The model under review builds one solid part; all positions refer to its coordinate system, in mm. Give positions to 0.01 mm unless a question says otherwise; leave off trailing zeros. Order: outer loops, then holes, each group sorted by start corner. A loop starts at its lowest first (then second) coordinate and runs counter-clockwise, first axis right, second up. Notation, with made-up numbers: (80.25, 50.5) -> (113.25, 50.5) arc R36 ccw to (113.25, 88.5) -> close; hole circle Ø9 at (-29, -3). An arc over 180 degrees is marked (long way). Use one line per item in the form item = value.
```python
from build123d import *

# Parameters (mm, degrees)
SKETCH1_W            = 20.32
SKETCH1_H            = 15.24
BOSS_EXTRUDE1_DEPTH  = 1.651
SKETCH3_W            = 3.048
SKETCH3_H            = 3.81
BOSS_EXTRUDE3_DEPTH  = 0.6604
SKETCH4_R            = 1.524
BOSS_EXTRUDE4_DEPTH  = 0.7366
SKETCH7_R            = 0.3937
CUT_EXTRUDE2_DEPTH   = 2.651
LPATTERN2_COUNT      = 8
LPATTERN2_PITCH      = 2.54
LPATTERN2_COUNT_DIR2 = 2
LPATTERN2_PITCH_DIR2 = 12.7
CUT_EXTRUDE3_REACH   = 3.651
SKETCH8_R            = 0.3937


with BuildPart() as part:
    # Sketch1 → Boss-Extrude1 (new body)
    with BuildSketch(Plane(origin=(0, 0, 0), x_dir=(1, 0, 0), z_dir=(0, 1, 0))):
        Rectangle(SKETCH1_W, SKETCH1_H)
    extrude(amount=BOSS_EXTRUDE1_DEPTH)

    # Sketch3 → Boss-Extrude3 (add)
    with BuildSketch(Plane(origin=(0, 1.651, 0), x_dir=(1, 0, 0), z_dir=(0, 1, 0))):
        with Locations((7.62, -2.921)):
            Rectangle(SKETCH3_W, SKETCH3_H)
    extrude(amount=BOSS_EXTRUDE3_DEPTH)

    # Sketch4 → Boss-Extrude4 (add)
    with BuildSketch(Plane(origin=(0, 2.3114, 0), x_dir=(1, 0, 0), z_dir=(0, 1, 0))):
        with Locations((7.62, -2.921)):
            Circle(SKETCH4_R)
        Polygon((7.8105, -2.7305), (8.636, -2.7305), (8.636, -3.1115), (7.8105, -3.1115), (7.8105, -3.937), (7.4295, -3.937), (7.4295, -3.1115), (6.604, -3.1115), (6.604, -2.7305), (7.4295, -2.7305), (7.4295, -1.905), (7.8105, -1.905), align=None, mode=Mode.SUBTRACT)
    extrude(amount=BOSS_EXTRUDE4_DEPTH)

    # Sketch7 → Cut-Extrude2 (cut, through all)
    with BuildSketch(Plane(origin=(0, 1.651, 0), x_dir=(1, 0, 0), z_dir=(0, 1, 0))):
        with Locations((-8.89, -6.35)):
            Circle(SKETCH7_R)
    cut_extrude2 = extrude(amount=-CUT_EXTRUDE2_DEPTH, mode=Mode.SUBTRACT)

    # LPattern2: Cut-Extrude2 8 × 2
    with Locations(*[(i * LPATTERN2_PITCH, 0, -j * LPATTERN2_PITCH_DIR2) for i in range(LPATTERN2_COUNT) for j in range(LPATTERN2_COUNT_DIR2) if (i, j) != (0, 0)]):
        add(cut_extrude2, mode=Mode.SUBTRACT)

    # Sketch8 → Cut-Extrude3 (cut, up to next)
    with BuildSketch(Plane(origin=(0, 1.651, 0), x_dir=(1, 0, 0), z_dir=(0, 1, 0)), mode=Mode.PRIVATE) as cut_extrude3_sk1:
        with Locations((8.89, 3.81)):
            Circle(SKETCH8_R)
    cut_extrude3_tool1 = extrude(cut_extrude3_sk1.sketch, amount=-CUT_EXTRUDE3_REACH, mode=Mode.PRIVATE) & part.part
    add(cut_extrude3_tool1.solids().sort_by_distance((8.89, 1.651, -3.81))[0], mode=Mode.SUBTRACT)
    # Sketch8 → Cut-Extrude3 (cut, up to next)
    with BuildSketch(Plane(origin=(0, 1.651, 0), x_dir=(1, 0, 0), z_dir=(0, 1, 0)), mode=Mode.PRIVATE) as cut_extrude3_sk2:
        with Locations((8.89, 1.27)):
            Circle(SKETCH8_R)
    cut_extrude3_tool2 = extrude(cut_extrude3_sk2.sketch, amount=-CUT_EXTRUDE3_REACH, mode=Mode.PRIVATE) & part.part
    add(cut_extrude3_tool2.solids().sort_by_distance((8.89, 1.651, -1.27))[0], mode=Mode.SUBTRACT)


solid = part.part
```
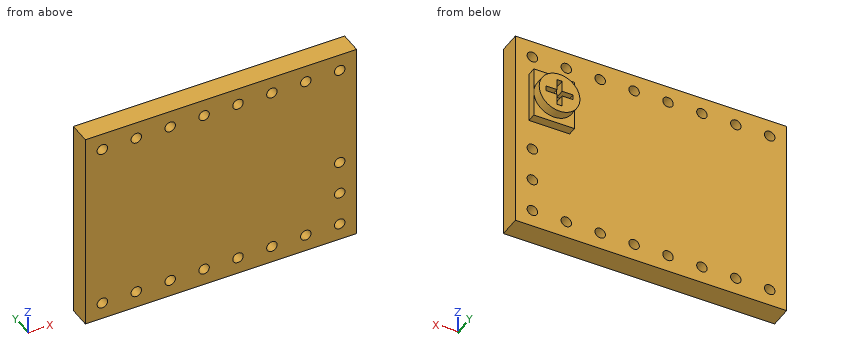
1. Add section A-A on z = -3.81. Give the boundary of the cut face in (x, y).
Values:
outline = (-10.16, 0) -> (8.5, 0) -> (8.5, 1.65) -> (-10.16, 1.65) -> close; (9.28, 0) -> (10.16, 0) -> (10.16, 1.65) -> (9.28, 1.65) -> close
2. Add section C-C on y = 0.35. Count the separate pieces of the cut face and the enclosed holes in it, then the cut area to 3 significant figures.
Values:
separate_pieces = 1
enclosed_holes = 18
area = 301 mm^2
3. For pin 1 Ø4 at (x, z) = (-7.5, 6) entering from -Y; pin 2 Ø0.5 at (y, z) = (2, 3) entering from -X; pin 3 Ø0.6 at (x, y) = (7, 2.5) entering from -Z; pin 4 Ø0.5 at (x, y) = (7.5, 2) entering from +Z, all flat-tipped, find the tip position at first contact; note any pin that passes through.
Values:
pin_1 = 0
pin_2 = 6.1
pin_3 = 1.02
pin_4 = 4.83
4. For L1, parallel to Z at x = 8.89, y = 0.55; L2, parallel to Z at x = 1.27, y = 0.9; L3, parallel to Y at x = -8.5, z = 3.5, list the stretches that pass through material, from the lowest coordinate up.
Values:
L1 = -7.62 to -6.74, -5.96 to -4.2, -3.42 to -1.66, -0.88 to 5.96, 6.74 to 7.62
L2 = -7.62 to -6.74, -5.96 to 5.96, 6.74 to 7.62
L3 = 0 to 1.65
5. Add section B-B on x = -8.89. Give the boundary of the cut face in (y, z), then the cut area to 3 significant figures.
Values:
outline = (0, -7.62) -> (1.65, -7.62) -> (1.65, -6.74) -> (0, -6.74) -> close; (0, -5.96) -> (1.65, -5.96) -> (1.65, 5.96) -> (0, 5.96) -> close; (0, 6.74) -> (1.65, 6.74) -> (1.65, 7.62) -> (0, 7.62) -> close
area = 22.6 mm^2
6. Add section D-D on x = 8.89. Give the boundary of the cut face in (y, z), then the cut area to 3 significant figures.
Values:
outline = (0, -7.62) -> (1.65, -7.62) -> (1.65, -6.74) -> (0, -6.74) -> close; (0, -5.96) -> (1.65, -5.96) -> (1.65, -4.2) -> (0, -4.2) -> close; (0, -3.42) -> (1.65, -3.42) -> (1.65, -1.66) -> (0, -1.66) -> close; (0, -0.88) -> (1.65, -0.88) -> (1.65, 1.02) -> (2.31, 1.02) -> (2.31, 2.08) -> (3.05, 2.08) -> (3.05, 3.76) -> (2.31, 3.76) -> (2.31, 4.83) -> (1.65, 4.83) -> (1.65, 5.96) -> (0, 5.96) -> close; (0, 6.74) -> (1.65, 6.74) -> (1.65, 7.62) -> (0, 7.62) -> close
area = 23.7 mm^2
